Geometry: see drawing. Coordinates: mm, zero at the bounding-box minimum. Coordinates: 2 decimals unless noted, no trailing zeros. Write each loop counter-clockwise with the first axis right and the second up, starting at its lowest first coordinate (ties: lowest second). Pieces come first, ordered by that corner, then holes. Notation, with made-up numbers: (11.5, -8) - (35.5, -8) arc R16 ccw to (35.5, 19) - close; hole circle Ø3 at (81, -40). An arc over 180 degrees is marked (long way). Use CSV: the item, a comma, the result in double quotes.
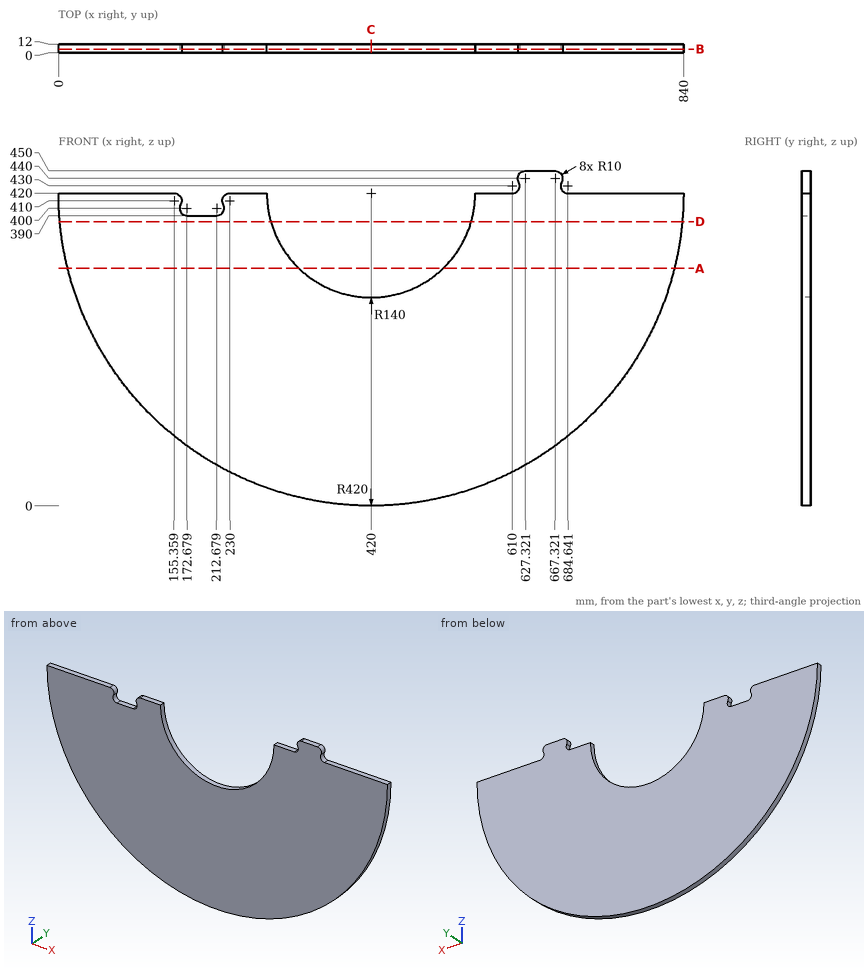
(1) Cut plane D-D on z = 382. Return loops of the section in (x, y) (1 decimal).
Check values:
outline,"(1.7, 0) - (285.3, 0) - (285.3, 12) - (1.7, 12) - close; (554.7, 0) - (838.3, 0) - (838.3, 12) - (554.7, 12) - close"
(2) Cut plane C-C on x = 420. Return loops of the section in (y, z), and give its area (3 significant figures).
Check values:
outline,"(0, 0) - (12, 0) - (12, 280) - (0, 280) - close"
area,"3,360 mm^2"
(3) Pin query (flat end, axial travel): pin 1 Ø6 at (y, z) = (10.5, 314) entering from -X (1 decimal); pin 2 Ø3.5 at (x, y) = (61.5, 3.5) entering from +Z; pin 3 Ø1.5 at (x, y) = (143.5, 7) entering from -Z. Return the tip coordinate at first contact, or that it passes through.
Check values:
pin 1,"x = 12.8"
pin 2,"z = 420"
pin 3,"z = 103.2"
(4) Cut plane A-A on z = 319. Return loops of the section in (x, y) (1 decimal), and give its area (3 significant figures).
Check values:
outline,"(12.3, 0) - (323.1, 0) - (323.1, 12) - (12.3, 12) - close; (516.9, 0) - (827.7, 0) - (827.7, 12) - (516.9, 12) - close"
area,"7,460 mm^2"
(5) Cut plane B-B on y = 5. Return loops of the section in (x, z).
Check values:
outline,"(0, 420) arc R420 ccw to (840, 420) - (684.64, 420) arc R10 cw to (675.98, 435) arc R10 ccw to (667.32, 450) - (627.32, 450) arc R10 ccw to (618.66, 435) arc R10 cw to (610, 420) - (560, 420) arc R140 cw to (280, 420) - (230, 420) arc R10 ccw to (221.34, 405) arc R10 cw to (212.68, 390) - (172.68, 390) arc R10 cw to (164.02, 405) arc R10 ccw to (155.36, 420) - close"
(6) Ray query, probe 1 along X at (y, z) = (11.25, 402) (1 decimal); probe 2 along X at (y, z) = (5.5, 406) (1 decimal); probe 3 along X at (y, z) = (9.5, 369). Return the intervals inside material, ascending. Write a range as from..to.
Check values:
probe 1,"0.4..162.9, 222.5..281.2, 558.8..839.6"
probe 2,"0.2..164.5, 220.8..280.7, 559.3..839.8"
probe 3,"3.11..289.62, 550.38..836.89"
